from build123d import *

# Parameters (mm, degrees)
SKETCH1_R             = 3.2639
BOSS_EXTRUDE1_DEPTH   = 12.7
CHAMFER1_SIZE         = 4.0894
CHAMFER1_SIZE2        = 3.554861186
CHAMFER1_PART_2_SIZE  = 4.0894
CHAMFER1_PART_2_SIZE2 = 3.554861186
CUT_EXTRUDE1_DEPTH    = 13.7000001


with BuildPart() as part:
    # Sketch1 → Boss-Extrude1 (new body)
    with BuildSketch(Plane(origin=(0, 0, 0), x_dir=(1, 0, 0), z_dir=(0, 1, 0))):
        with BuildLine():
            Line((-8.873253367, 0), (29.595519551, 0))
            add(Edge.make_bspline(
                [(29.595519551, 0), (32.608022391, -14.845023466), (66.17675893, -13.698872415), (72.627485997, 5.074574194)],
                knots=[0, 0, 0, 0, 1, 1, 1, 1], degree=3))
            Line((72.627485997, 5.074574194), (76.972410672, -0.328799158))
            ThreePointArc((76.972410672, -0.328799158), (56.487992256, -17.897771795), (30.865519551, -26.369435729))
            Line((30.865519551, -26.369435729), (18.165519551, -18.896027316))
            Line((18.165519551, -18.896027316), (-5.688817186, -18.896027316))
            ThreePointArc((-5.688817186, -18.896027316), (-18.253794481, -13.20459823), (-29.23375861, -4.855262498))
            Line((-29.23375861, -4.855262498), (-29.23375861, 4.177286104))
            ThreePointArc((-29.23375861, 4.177286104), (-28.489809834, 5.973337328), (-26.69375861, 6.717286104))
            Line((-26.69375861, 6.717286104), (-16.191261416, 6.717286104))
            ThreePointArc((-16.191261416, 6.717286104), (-15.013419953, 6.427683732), (-14.10416564, 5.624915621))
            Line((-14.10416564, 5.624915621), (-10.960349143, 1.092370482))
            ThreePointArc((-10.960349143, 1.092370482), (-10.05109483, 0.289602371), (-8.873253367, 0))
        make_face()
        with Locations((-20.368787798, -1.624222444)):
            Circle(SKETCH1_R, mode=Mode.SUBTRACT)
        with Locations((-7.908365266, -9.317144856)):
            Circle(SKETCH1_R, mode=Mode.SUBTRACT)
        with Locations((7.107001098, -10.503835127)):
            Circle(SKETCH1_R, mode=Mode.SUBTRACT)
        with Locations((22.444824189, -11.767482364)):
            Circle(SKETCH1_R, mode=Mode.SUBTRACT)
    extrude(amount=BOSS_EXTRUDE1_DEPTH)

    # Chamfer1
    chamfer1_edges = [part.edges().sort_by_distance(p)[0] for p in [
        (-23.632687798, 12.7, 1.624222444),
    ]]
    chamfer1_side = [part.faces().sort_by_distance(p)[0] for p in [
        (-23.632687798, 6.35, 1.624222444),
    ]]
    chamfer(chamfer1_edges, length=CHAMFER1_SIZE, length2=CHAMFER1_SIZE2, reference=chamfer1_side[0])

    # Chamfer1 part 2
    chamfer1_part_2_edges = [part.edges().sort_by_distance(p)[0] for p in [
        (3.843101098, 12.7, 10.503835127),
    ]]
    chamfer1_part_2_side = [part.faces().sort_by_distance(p)[0] for p in [
        (3.843101098, 6.35, 10.503835127),
    ]]
    chamfer(chamfer1_part_2_edges, length=CHAMFER1_PART_2_SIZE, length2=CHAMFER1_PART_2_SIZE2, reference=chamfer1_part_2_side[0])

    # Sketch2 → Cut-Extrude1 (cut, through all)
    with BuildSketch(Plane(origin=(0, 12.7, 0), x_dir=(1, 0, 0), z_dir=(0, 1, 0))):
        Polygon((-2.191584648, -6.154850089), (-7.78860256, -2.78512023), (-13.505383178, -5.947414997), (-13.625145885, -12.479439623), (-8.028127973, -15.849169483), (-2.311347355, -12.686874716), align=None)
        Polygon((28.471794253, -14.28885514), (27.641882098, -7.808659569), (21.614912034, -5.287286792), (16.417854125, -9.246109587), (17.247766281, -15.726305159), (23.274736345, -18.247677935), align=None)
    extrude(amount=-CUT_EXTRUDE1_DEPTH, mode=Mode.SUBTRACT)


solid = part.part
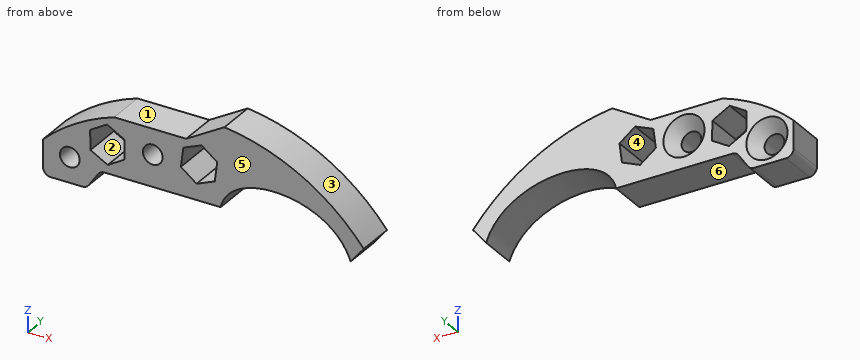
Part model, mm, in its own coordinate system. Face numbers are marked on the shaded views. A direction names the side the tool comes from. Give positions to 0.01 mm unless a question says otherwise; leave off trailing zeros.
1) Which spindle directions (+Z, -Z, +X, -X, +Y, -Y) get a long thin tool onto all of the face, cutting with end or side? Do the marked faces 4, 5 and 6. Say none if no direction does.
Resolved:
face 4: +Y, -Y
face 5: +Z, -Z, +X, -X, -Y
face 6: -Z, +Y, -Y
2) Cut at A-A on y = 7.25. State how many separate pieces and enclosed holes the cut face has, then the cut area to 3 significant figures.
Resolved:
separate pieces: 1
enclosed holes: 4
area: 1,380 mm2
3) Two-plate mould, pull along X, no slides. Class the marked faces 1, 2 and 3: released by +X, released by -X, zero draft, split by the parting line, or undercut.
Resolved:
face 1: zero draft
face 2: undercut
face 3: released by +X
4) Pin check, flat tips, straight feed: pin 1 (1.5 mm diameter, centred on x = -4, y = 6.5, fed in from -Z); pin 2 (6 mm diameter, centred on x = 7.11, z = 10.5, fed in from +Y); pin 3 (7.5 mm diameter, centred on x = -20.37, z = 1.62, fed in from +Y); pin 4 (1 mm diameter, centred on x = 59, y = 6, fed in from -Z). Stop position of each tip, or through.
Resolved:
pin 1: stops at z = 0
pin 2: passes through
pin 3: stops at y = 9.17
pin 4: stops at z = 7.79
5) Probe L1, parallel to X at y = 10.25, z = 2; L2, parallel to X at y = 2, z = 5.5; L3, parallel to X at y = 11.5, z = 0.5. List the from-to ranges inside material, lowest first.
Resolved:
L1: x = -29.23 to -25.04, -15.69 to 30.22, 68.27 to 75.61
L2: x = -28.55 to -12.7, -3.28 to 21.34, 22.12 to 32.72, 63.97 to 72.47
L3: x = -29.23 to -26.03, -14.7 to 29.71, 69.58 to 76.84
